The model under review builds one solid part; all positions refer to its coordinate system, in mm. A direction names the side the tool comes from. Give positions to 0.01 mm unless a question says otherwise; leave off trailing zeros. Order: outer loops, then holes, each group sorted by start corner. A loop starts at its lowest first (then second) coordinate and runs counter-clockwise, first axis right, second up. Notation, with made-up numbers: (-1, 81.25) -> (29, 81.25) arc R26 cw to (29, 116.25) -> close; hole circle Ø4 at (-33.5, -29). An arc over 180 degrees is marked (long way). Use one line per item in the form item = value.
```python
from build123d import *

# Parameters (mm, degrees)
F0_R           = 2.75
F1_DEPTH       = 18.5
F3_DEPTH       = 8
F7_D           = 2
F7_DEPTH       = 6
F7_TIP         = 0.600860619
F7_ON_F5_D     = 2
F7_ON_F5_DEPTH = 6
F7_ON_F5_TIP   = 0.600860619
F8_R           = 0.2


with BuildPart() as f1:
    # F0 (on Front) → F1 (new body, symmetric)
    with BuildSketch(Plane.XZ):
        Circle(F0_R)
    extrude(amount=F1_DEPTH, both=True)

    # F2 (on face) → F3 (cut)
    with BuildSketch(Plane.XZ.offset(18.5)):
        with BuildLine():
            ThreePointArc((1.9880895352, 1.9), (1.0810874155, 2.5285865617), (0, 2.75))
            ThreePointArc((0, 2.75), (-1.0810874155, 2.5285865617), (-1.9880895352, 1.9))
            Line((-1.9880895352, 1.9), (1.9880895352, 1.9))
        make_face()
        with BuildLine():
            Line((1.9880895352, -1.9), (-1.9880895352, -1.9))
            ThreePointArc((-1.9880895352, -1.9), (-1.0810874155, -2.5285865617), (0, -2.75))
            ThreePointArc((0, -2.75), (1.0810874155, -2.5285865617), (1.9880895352, -1.9))
        make_face()
    extrude(amount=-F3_DEPTH, mode=Mode.SUBTRACT)

    # F4: F1 across plane


with BuildPart() as f1_1:
    add(f1.part)
    add(f1.part.mirror(Plane.XZ), mode=Mode.INTERSECT)

    # F7
    with Locations(Plane(origin=(0, 18.5, 0), x_dir=(-1, 0, 0), z_dir=(0, 1, 0))):
        with Locations((0, 0)):
            Hole(F7_D / 2, depth=F7_DEPTH)
            with Locations((0, 0, -(F7_DEPTH + F7_TIP / 2))):  # 118° drill point
                Cone(0, F7_D / 2, F7_TIP, mode=Mode.SUBTRACT)

    # F7 on F5
    with Locations(Plane.XZ.offset(18.5)):
        with Locations((0, 0)):
            Hole(F7_ON_F5_D / 2, depth=F7_ON_F5_DEPTH)
            with Locations((0, 0, -(F7_ON_F5_DEPTH + F7_ON_F5_TIP / 2))):  # 118° drill point
                Cone(0, F7_ON_F5_D / 2, F7_ON_F5_TIP, mode=Mode.SUBTRACT)

    # F8
    f8_edges = [f1_1.edges().sort_by_distance(p)[0] for p in [
        (2.552425, -18.5, 1.023536),
        (-2.75, -18.5, 0),
        (2.552425, -18.5, -1.023536),
        (-1.98809, -14.5, -1.9),
        (1.98809, -14.5, -1.9),
        (1.98809, -14.5, 1.9),
        (-1.98809, -14.5, 1.9),
        (0, -18.5, -1.9),
        (0, -18.5, 1.9),
        (1.98809, 14.5, 1.9),
        (-1.98809, 14.5, 1.9),
        (-1.98809, 14.5, -1.9),
        (1.98809, 14.5, -1.9),
        (2.552425, 18.5, -1.023536),
        (0, 18.5, -1.9),
        (2.552425, 18.5, 1.023536),
        (-2.75, 18.5, 0),
        (0, 18.5, 1.9),
        (1, 18.5, 0),
        (-1, -18.5, 0),
    ]]
    fillet(f8_edges, radius=F8_R)


solid = f1_1.part
```
1. Add section B-B on z = 2.25. Give the boundary of the cut face in (x, y), then the cut area to 3 significant figures.
Values:
outline = (-1.58, -10.5) -> (1.58, -10.5) -> (1.58, 10.5) -> (-1.58, 10.5) -> close
area = 66.4 mm^2
2. Add section A-A on y = 0.5. Give the boundary of the cut face in (x, z), then the cut area to 3 significant figures.
Values:
outline = circle Ø5.5 at (0, 0)
area = 23.8 mm^2
3. For pin 1 Ø1 at (y, z) = (11, 2) entering from +X; pin 2 Ø0.5 at (x, z) = (0, 2.5) entering from -Y; pin 3 Ø3 at (x, y) = (0, -13) entering from +Z, all flat-tipped, find the tip position at first contact; note any pin that passes through.
Values:
pin_1 = 2.3
pin_2 = -10.5
pin_3 = 1.9
4. The part is to be moulded in two halves that separate along X. For faces 6 (the face through (0, 15, -1)), 7 (the face through (-0.596, -0.256, -2.685)), 8 (the face through (0, -14, -1.9)), 9 (the face through (0, -15, -1)), say which applies: +X half, -X half, draft (parallel to the pull), parting line (faces both ways), or undercut.
Values:
face_6 = undercut
face_7 = parting line
face_8 = draft
face_9 = undercut
5. Tool access review of faces 1 (the face through (0, 14, 1.9)), 2 (the face through (1, 18.5, 1)), 3 (the face through (1, -18.5, 1)), 4 (the face through (0, 14, -1.9)), 5 (the face through (0, -14, 1.9)): name each direction out of +Z, -Z, +X, -X, +Y, -Y from which nothing blocks a thin tool from reaching the whole face with its end or side.
Values:
face_1 = +Z, +X, -X, +Y
face_2 = +Z, -Z, +X, -X, +Y
face_3 = +Z, -Z, +X, -X, -Y
face_4 = -Z, +X, -X, +Y
face_5 = +Z, +X, -X, -Y
6. For L1, parallel to Z at x = 0, y = -16.35; L2, parallel to X at y = 15.6, z = 0; L3, parallel to Z at x = -0.9, y = 11.5, list the stretches that pass through material, from the lowest coordinate up.
Values:
L1 = -1.9 to -1, 1 to 1.9
L2 = -2.75 to -1, 1 to 2.75
L3 = -1.9 to 1.9
